Design review of the part shown in the three views and the two pictorial views. Dimensions are in mm from the part's minimum x, y and z. A direction names the side the tool comes from. Round coordinates to 2 decimals unless told otherwise and drop trailing zeros. Order: outer loops, then holes, each group sorted by start corner. A loop starts at its lowest first (then second) coordinate and runs counter-clockwise, first axis right, second up.
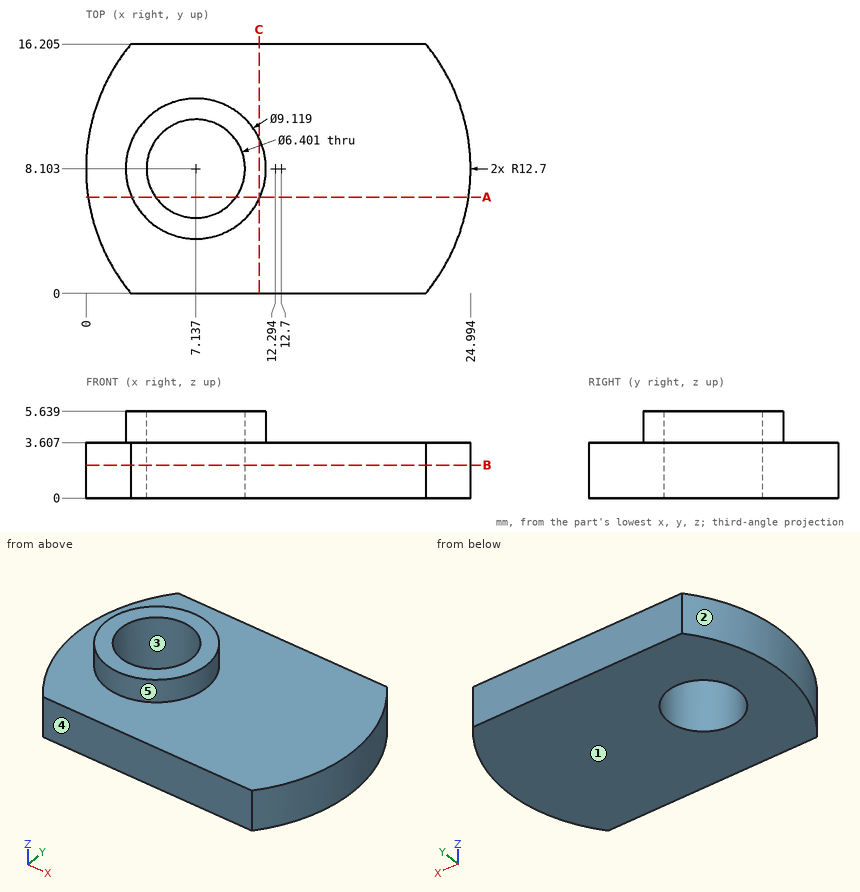
(1) Add section A-A on y = 6.25. Give the boundary of the cut face in (x, z).
(2) Wall thickness on L1, parallel to X at y = 8.25, z = 0.95 (1 decimal); L2, parallel to Z at x = 16.75, y = 9.25; L3, parallel to Y at x = 8.75, z = 5.3: over which ranges is each line inside the solid? List them lowest first.
(3) Add section B-B on z = 2.15. Give the boundary of the cut face in (x, y) (1 decimal), plus the area to 3 significant figures.
(4) Clearance check with a flat-ended pin moving along its axis: P1, Ø1.5, axis at x = 11.5, y = 5, coming from the +Z side. State where the tip first meets the part, or that it passes through.
(5) Add section C-C on x = 11.25. Give the boundary of the cut face in (y, z) (1 decimal).
(6) Tool access review of the marked faces 4 and 5: name each direction out of +Z, -Z, +X, -X, +Y, -Y from which nothing blocks a thin tool from reaching the whole face with its end or side.
(7) Draft analysis for pull direction X (two halves, no side actions). For the marked faces 1, 2 and 3, state which applies: pulls with the +X half, pulls with the -X half, needs draft (parallel to the pull), parting line crosses it, or undercut.
Here are the results:
1. outline: (0.14, 0) - (4.53, 0) - (4.53, 5.64) - (2.97, 5.64) - (2.97, 3.61) - (0.14, 3.61) - close; (9.75, 0) - (24.86, 0) - (24.86, 3.61) - (11.3, 3.61) - (11.3, 5.64) - (9.75, 5.64) - close
2. L1: x = 0 to 3.9, 10.3 to 25
2. L2: z = 0 to 3.61
2. L3: y = 3.84 to 5.34, 10.87 to 12.37
3. outline: (2.9, 0) - (22.1, 0) arc R12.7 ccw to (22.1, 16.2) - (2.9, 16.2) arc R12.7 ccw to start; hole circle Ø6.4 at (7.1, 8.1)
3. area: 343 mm2
4. P1: stops at z = 3.61
5. outline: (0, 0) - (16.2, 0) - (16.2, 3.6) - (10.1, 3.6) - (10.1, 5.6) - (6.1, 5.6) - (6.1, 3.6) - (0, 3.6) - close
6. face 4: +Z, -Z, +X, -X, -Y
6. face 5: +Z
7. face 1: needs draft
7. face 2: pulls with the -X half
7. face 3: undercut
